Check sheet for the modelled part. Datum: model origin and axes. Units: mm. A direction names the side the tool comes from. Give positions to 0.01 mm unless a question says otherwise; leave off trailing zeros. Write each loop counter-clockwise with the first axis right and the second up, starting at its lowest first coordinate (ties: lowest second). Pieces come first, ordered by that corner, then holes.
from build123d import *

# Parameters (mm, degrees)
BOSS_EXTRUDE1_DEPTH      = 21.25
BOSS_EXTRUDE1_DEPTH_BACK = 21.25
SKETCH2_R                = 2
CUT_EXTRUDE1_DEPTH       = 140.683794694
SKETCH3_W                = 82
SKETCH3_H                = 127.094201992
BOSS_EXTRUDE2_DEPTH      = 52


with BuildPart() as part:
    # Sketch1 → Boss-Extrude1 (new, two sides: drawn at the far end of the back side and taken through both)
    with BuildSketch(Plane(origin=(0, 0, 0), x_dir=(1, 0, 0), z_dir=(0, 1, 0)).offset(-BOSS_EXTRUDE1_DEPTH_BACK)):
        Polygon((-43, -22), (-35, 0), (35, 0), (43, -22), (43, -108), (-43, -108), align=None)
    extrude(amount=BOSS_EXTRUDE1_DEPTH + BOSS_EXTRUDE1_DEPTH_BACK)

    # Sketch2 → Cut-Extrude1 (cut, through all)
    with BuildSketch(Plane(origin=(43, 0, 0), x_dir=(0, 0, -1), z_dir=(1, 0, 0))):
        with Locations((-71.25, 9.2)):
            Circle(SKETCH2_R)
        with Locations((-42.75, 9.2)):
            Circle(SKETCH2_R)
        with Locations(Location((-42.75, -9.2, 0), (0, 0, 180))):
            Circle(SKETCH2_R)
        with Locations(Location((-71.25, -9.2, 0), (0, 0, 180))):
            Circle(SKETCH2_R)
    extrude(amount=-CUT_EXTRUDE1_DEPTH, mode=Mode.SUBTRACT)

    # Sketch3 → Boss-Extrude2 (add)
    with BuildSketch(Plane(origin=(0, 21.25, 0), x_dir=(1, 0, 0), z_dir=(0, 1, 0))):
        with Locations((0, -48.227100996)):
            Rectangle(SKETCH3_W, SKETCH3_H)
    boss_extrude2 = extrude(amount=BOSS_EXTRUDE2_DEPTH)

    # Mirror1: Boss-Extrude2 across plane
    add(boss_extrude2.mirror(Plane.ZX))


solid = part.part
1) Draft check along Z on faces 1 (the flat face through (43, 0, 64)), 2 (the cylindrical face through (0.602, -10.552, 41.276)), 3 (the flat face through (-1, 47, 111.774)). Enter one of: +Z half, -Z half, draft (parallel to the pull), parting line (faces both ways), or undercut.
2) Sectioned sample at B-B on y = 9.2. Record the boundary of the cut face in (x, z).
3) Sectioned sample at D-D on z = 31. Record the boundary of the cut face in (x, y).
4) Sectioned sample at A-A on z = 71.25. Record the boundary of the cut face in (x, y), then the cut area to 3 significant figures.
5) Scan lines: L1, parallel to Z at x = -4, y = 9; L2, parallel to Y at x = 6, z = 42; L3, parallel to X at y = 40, z = 42.5. Record each from-to range of solid material in increasing order.
6) Access from +Z, -Z, +X, -X, +Y, -Y to the whole of each face (thin tool, end or side, straight path). Record for faces 4 (the flat face through (-1, -21.25, 110)), 5 (the flat face through (-39, 0, 11)), 6 (the flat face through (0, 0, 0)), 7 (the flat face through (41, 47, 49)), 8 (the flat face through (39, 0, 11)).
7) Sectioned sample at C-C on x = 17.5. Record the boundary of the cut face in (y, z), then the cut area to 3 significant figures.
8) Gauge pin test, flat ends, axial feed: pin 1 (0.6 mm diameter, centred on x = 42, z = 45, fed in from +Y); pin 2 (1 mm diameter, centred on x = -17.5, y = 13.5, fed in from -Z); pin 3 (3 mm diameter, centred on y = -9.2, z = 71.25, fed in from +X); pin 4 (6 mm diameter, centred on y = 30, z = 29, fed in from -X). Record the tip position at first contact, or that the pin passes through.
Answers below:
1. face 1: draft
1. face 2: undercut
1. face 3: +Z half
2. outline: (-43, 22) - (-35, 0) - (35, 0) - (43, 22) - (43, 40.75) - (-43, 40.75) - close; (-43, 44.75) - (43, 44.75) - (43, 69.25) - (-43, 69.25) - close; (-43, 73.25) - (43, 73.25) - (43, 108) - (-43, 108) - close
3. outline: (-43, -21.25) - (-41, -21.25) - (-41, -73.25) - (41, -73.25) - (41, -21.25) - (43, -21.25) - (43, 21.25) - (41, 21.25) - (41, 73.25) - (-41, 73.25) - (-41, 21.25) - (-43, 21.25) - close
4. outline: (-43, -21.25) - (-41, -21.25) - (-41, -73.25) - (41, -73.25) - (41, -21.25) - (43, -21.25) - (43, -11.2) - (-43, -11.2) - close; (-43, -7.2) - (43, -7.2) - (43, 7.2) - (-43, 7.2) - close; (-43, 11.2) - (43, 11.2) - (43, 21.25) - (41, 21.25) - (41, 73.25) - (-41, 73.25) - (-41, 21.25) - (-43, 21.25) - close
4. area: 11,500 mm2
5. L1: z = 0 to 40.76, 44.74 to 69.26, 73.24 to 108
5. L2: y = -73.25 to -11.05, -7.35 to 7.35, 11.05 to 73.25
5. L3: x = -41 to 41
6. face 4: +Z, +X, -X
6. face 5: -Z, -X
6. face 6: -Z, +X, -X
6. face 7: +Z, -Z, +X, +Y
6. face 8: -Z, +X
7. outline: (-73.25, -15.32) - (-21.25, -15.32) - (-21.25, 0) - (21.25, 0) - (21.25, -15.32) - (73.25, -15.32) - (73.25, 111.77) - (21.25, 111.77) - (21.25, 108) - (-21.25, 108) - (-21.25, 111.77) - (-73.25, 111.77) - close; hole circle Ø4 at (-9.2, 42.75); hole circle Ø4 at (-9.2, 71.25); hole circle Ø4 at (9.2, 42.75); hole circle Ø4 at (9.2, 71.25)
7. area: 17,800 mm2
8. pin 1: stops at y = 21.25
8. pin 2: stops at z = 0
8. pin 3: passes through
8. pin 4: stops at x = -41
